Build history of the part. All positions in model axes, mm. A direction names the side the tool comes from. Round coordinates to 2 decimals unless told otherwise and drop trailing zeros. Write each loop counter-clockwise with the first axis right and the second up, starting at its lowest first coordinate (ties: lowest second). Pieces come first, ordered by that corner, then holes. Notation, with made-up numbers: M -27.5,63.25 L 12.5,63.25 A24 cw 12.5,76.25 Z; hole C 2,32.5 d11. An arc over 180 degrees is marked long. Write item = value, one per line. Start each with the question number.
Q1. Band-saw the part on D-D on z = -40.5. Write the cut outline in (x, y), plus the area to 3 significant figures.
Q2. Tool access for faces 1 (the flat face through (9, 0, 1)), 2 (the cylindrical face through (-1.075, -9.493, 66.686)): list every direction of +Z, -Z, +X, -X, +Y, -Y with a clear straight run to the whole face (end or side of a thin tool).
Q3. Band-saw the part on B-B on z = 8.5. Write the cut outline in (x, y), plus the area to 3 significant figures.
Q4. Band-saw the part on A-A on x = -5. Write the cut outline in (y, z), plus the area to 3 significant figures.
Q5. Probe L1, parallel to Y at x = -5.25, z = 85. List the from-to ranges inside material, lowest first.
Q6. Pull direction X, two halves, no side cores. Call faces 3 (the cylindrical face through (0.26, 9.507, 10.483)), 4 (the cylindrical face through (-0.923, 9.507, 48.226)), 5 (the flat face through (-10, 0, 1)), 6 (the flat face through (-0.8, -9.6, 105)): released by +X, released by -X, zero draft, split by the parting line, or undercut.
```python
from build123d import *

# Parameters (mm, degrees)
SKETCH_1_W          = 20
SKETCH_1_H          = 20
SKETCH_1_W_2        = 18
SKETCH_1_H_2        = 18
EXTRUDE_1_DEPTH     = 105
SKETCH_2_R          = 2
CUT_EXTRUDE_1_DEPTH = 108.354552768
SKETCH_3_R          = 2
CUT_EXTRUDE_2_DEPTH = 108.354552768


with BuildPart() as part:
    # 草图1 → 凸台-拉伸1 (new, symmetric)
    with BuildSketch(Plane.XY):
        Rectangle(SKETCH_1_W, SKETCH_1_H)
        Rectangle(SKETCH_1_W_2, SKETCH_1_H_2, mode=Mode.SUBTRACT)
    extrude(amount=EXTRUDE_1_DEPTH, both=True)

    # 草图2 → 切除-拉伸1 (cut, through all)
    with BuildSketch(Plane(origin=(0, 10, 0), x_dir=(1, 0, 0), z_dir=(0, 1, 0))):
        with Locations(Location((0, 65, 0), (0, 0, 180))):
            Circle(SKETCH_2_R)
        with Locations(Location((0, -65, 0), (0, 0, 180))):
            Circle(SKETCH_2_R)
        with Locations(Location((0, -50, 0), (0, 0, 180))):
            Circle(SKETCH_2_R)
        with Locations(Location((0, 50, 0), (0, 0, 180))):
            Circle(SKETCH_2_R)
    extrude(amount=-CUT_EXTRUDE_1_DEPTH, mode=Mode.SUBTRACT)

    # 草图3 → 切除-拉伸2 (cut, through all)
    with BuildSketch(Plane(origin=(0, 10, 0), x_dir=(1, 0, 0), z_dir=(0, 1, 0))):
        with Locations(Location((0, -8.5, 0), (0, 0, 180))):
            Circle(SKETCH_3_R)
        with Locations(Location((0, 6.5, 0), (0, 0, 180))):
            Circle(SKETCH_3_R)
        with Locations(Location((0, -23.5, 0), (0, 0, 180))):
            Circle(SKETCH_3_R)
    extrude(amount=-CUT_EXTRUDE_2_DEPTH, mode=Mode.SUBTRACT)


solid = part.part
```
Conclusion:
q1.outline = M -10,-10 L 10,-10 L 10,10 L -10,10 Z; hole M -9,-9 L 9,-9 L 9,9 L -9,9 Z
q1.area = 76.0 mm^2
q2.face_1 = +Z, -Z
q2.face_2 = +Y, -Y
q3.outline = M -10,-10 L -2,-10 L -2,-9 L -9,-9 L -9,9 L -2,9 L -2,10 L -10,10 Z; M 2,-10 L 10,-10 L 10,10 L 2,10 L 2,9 L 9,9 L 9,-9 L 2,-9 Z
q3.area = 68.0 mm^2
q4.outline = M -10,-105 L -9,-105 L -9,105 L -10,105 Z; M 9,-105 L 10,-105 L 10,105 L 9,105 Z
q4.area = 420 mm^2
q5.L1 = -10 to -9, 9 to 10
q6.face_3 = undercut
q6.face_4 = undercut
q6.face_5 = released by -X
q6.face_6 = zero draft
